Build history of the part. All positions in model axes, mm. Face numbers are marked on the shaded views. A direction names the side the tool comes from. Round coordinates to 2 decimals unless told otherwise and drop trailing zeros. Write each loop counter-clockwise with the first axis right and the second up, starting at its lowest first coordinate (ties: lowest second). Pieces come first, ordered by that corner, then holes.
1) Which spindle directions (+Z, -Z, +X, -X, +Y, -Y) get a long thin tool onto all of the face, cutting with end or side? Do the marked faces 1 and 2. Say none if no direction does.
2) Saw through at D-D (x = 3.5). Write the cut outline in (y, z).
3) Pull direction X, two halves, no side cores. Call the marked faces 3, 4, 5 and 6: +X half, -X half, draft (parallel to the pull), parting line (faces both ways), or undercut.
4) Saw through at A-A (x = 26.5). Write the cut outline in (y, z).
5) Saw through at C-C (y = 15). Write the cut outline in (x, z), plus the area to 3 significant figures.
6) Saw through at B-B (z = 3.5). Write the cut outline in (x, y), plus the area to 3 significant figures.
7) Wall check: probe 1 along Y at (x, z) = (26.5, 2.25); probe 2 along Y at (x, z) = (13.25, 3.6); probe 3 along Y at (x, z) = (3.5, 1.9). Give the ranges that are in metal, low to high.
8) Flat gauge pin, fed straight in: pin 1 (1.8 mm diameter, centred on x = 26.5, y = 4.52, fed in from +Z). Where does the tip first touch, or does it go through?
from build123d import *

# Parameters (mm, degrees)
SKETCH_1_R               = 1.5
EXTRUDE_1_DEPTH          = 4
CUT_EXTRUDE_1_DEPTH      = 1
CUT_EXTRUDE_1_DEPTH_BACK = 4


with BuildPart() as part:
    # Эскиз1 → Бобышка-Вытянуть1 (new body)
    with BuildSketch(Plane.XY):
        with BuildLine():
            Line((0, 0), (30, 0))
            Line((30, 0), (30, 17.5))
            ThreePointArc((30, 17.5), (29.267766953, 19.267766953), (27.5, 20))
            Line((27.5, 20), (2.5, 20))
            ThreePointArc((2.5, 20), (0.732233047, 19.267766953), (0, 17.5))
            Line((0, 17.5), (0, 0))
        make_face()
        with Locations((3.5, 15)):
            Circle(SKETCH_1_R, mode=Mode.SUBTRACT)
        with Locations((26.5, 15)):
            Circle(SKETCH_1_R, mode=Mode.SUBTRACT)
        with Locations((26.5, 4.52)):
            Circle(SKETCH_1_R, mode=Mode.SUBTRACT)
    extrude(amount=EXTRUDE_1_DEPTH)

    # Эскиз2 → Вырез-Вытянуть1 (cut, two sides)
    with BuildSketch(Plane.XY.offset(4)) as cut_extrude_1_sk:
        Polygon((13.5, 5.25), (13.5, 0), (16.5, 0), (16.5, 5.25), (17.75, 5.25), (17.75, 7.75), (16.5, 7.75), (16.5, 13), (13.5, 13), (13.5, 7.75), (12.25, 7.75), (12.25, 5.25), align=None)
    extrude(amount=CUT_EXTRUDE_1_DEPTH, mode=Mode.SUBTRACT)
    extrude(cut_extrude_1_sk.sketch, amount=-CUT_EXTRUDE_1_DEPTH_BACK, mode=Mode.SUBTRACT)


solid = part.part
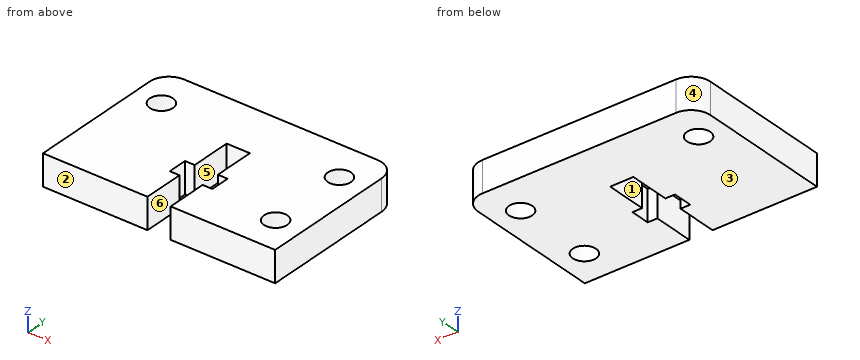
Evaluation:
1. face 1: +Z, -Z, -Y
1. face 2: +Z, -Z, +X, -X, -Y
2. outline: (0, 0) - (13.5, 0) - (13.5, 4) - (0, 4) - close; (16.5, 0) - (20, 0) - (20, 4) - (16.5, 4) - close
3. face 3: draft
3. face 4: -X half
3. face 5: undercut
3. face 6: undercut
4. outline: (0, 0) - (3.02, 0) - (3.02, 4) - (0, 4) - close; (6.02, 0) - (13.5, 0) - (13.5, 4) - (6.02, 4) - close; (16.5, 0) - (20, 0) - (20, 4) - (16.5, 4) - close
5. outline: (0, 0) - (2, 0) - (2, 4) - (0, 4) - close; (5, 0) - (25, 0) - (25, 4) - (5, 4) - close; (28, 0) - (30, 0) - (30, 4) - (28, 4) - close
5. area: 96.0 mm2
6. outline: (0, 0) - (13.5, 0) - (13.5, 5.25) - (12.25, 5.25) - (12.25, 7.75) - (13.5, 7.75) - (13.5, 13) - (16.5, 13) - (16.5, 7.75) - (17.75, 7.75) - (17.75, 5.25) - (16.5, 5.25) - (16.5, 0) - (30, 0) - (30, 17.5) arc R2.5 ccw to (27.5, 20) - (2.5, 20) arc R2.5 ccw to (0, 17.5) - close; hole circle Ø3 at (3.5, 15); hole circle Ø3 at (26.5, 4.52); hole circle Ø3 at (26.5, 15)
6. area: 531 mm2
7. probe 1: y = 0 to 3.02, 6.02 to 13.5, 16.5 to 20
7. probe 2: y = 0 to 5.25, 7.75 to 20
7. probe 3: y = 0 to 13.5, 16.5 to 20
8. pin 1: passes through
